Could you check a few things on this model? Use its own coordinates, in mm. Face numbers are marked on the shaded views. A direction names the side the tool comes from. Coordinates: 2 decimals unless noted, no trailing zeros. Write each loop counter-clockwise with the first axis right and the second up, starting at its lowest first coordinate (ties: lowest second). Pieces come first, ordered by that corner, then holes.
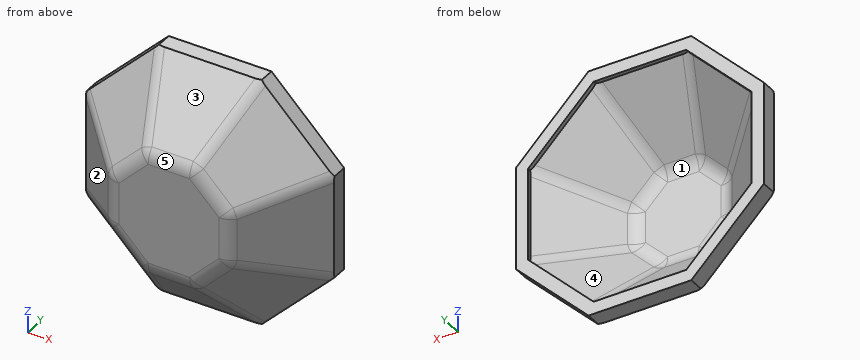
Autodesk Inventor part; units mm, degrees
ref_plane "YZ Plane" through (0, 0, 0) normal (1, 0, 0) x (0, 1, 0)
ref_plane "XZ Plane" through (0, 0, 0) normal (0, 1, 0) x (-1, 0, 0)
ref_plane "XY Plane" through (0, 0, 0) normal (0, 0, 1) x (1, 0, 0)
sketch "Sketch1" plane through (0, 0, 0) normal (0, 1, 0) x (-1, 0, 0)
  line L0 (-62.7534, -151.5) -> (-151.5, -62.7534)
  line L1 (-151.5, -62.7534) -> (-151.5, 62.7534)
  line L2 (-151.5, 62.7534) -> (-62.7534, 151.5)
  line L3 (-62.7534, 151.5) -> (62.7534, 151.5)
  line L4 (62.7534, 151.5) -> (151.5, 62.7534)
  line L5 (151.5, 62.7534) -> (151.5, -62.7534)
  line L6 (151.5, -62.7534) -> (62.7534, -151.5)
  line L7 (62.7534, -151.5) -> (-62.7534, -151.5)
  point P0 (0, 0)
  point P1 (0, 0)
  dimension "d0" = 303
extrude "Extrusion1" add sketch "Sketch1" along normal blind 100
sketch "Sketch2" plane through (0, 100, 0) normal (0, 1, 0) x (1, 0, 0)
  line L0 (-136.5, 56.5402) -> (-56.5402, 136.5)
  line L1 (-56.5402, 136.5) -> (56.5402, 136.5)
  line L2 (56.5402, 136.5) -> (136.5, 56.5402)
  line L3 (136.5, 56.5402) -> (136.5, -56.5402)
  line L4 (136.5, -56.5402) -> (56.5402, -136.5)
  line L5 (56.5402, -136.5) -> (-56.5402, -136.5)
  line L6 (-56.5402, -136.5) -> (-136.5, -56.5402)
  line L7 (-136.5, -56.5402) -> (-136.5, 56.5402)
  point P0 (0, 0)
  point P1 (0, 0)
  dimension "d3" = 273
extrude "Extrusion2" cut sketch "Sketch2" against normal blind 85
chamfer "Chamfer1" distance 80 angle 45 8 edges at (0, 15, 136.5) (96.5201, 15, 96.5201) (-96.5201, 15, 96.5201) (136.5, 15, 0) (96.5201, 15, -96.5201) (0, 15, -136.5) (-96.5201, 15, -96.5201) (-136.5, 15, 0)
chamfer "Chamfer2" distance 80 angle 45 8 edges at (-107.1267, 0, -107.1267) (0, 0, -151.5) (-151.5, 0, 0) (107.1267, 0, -107.1267) (151.5, 0, 0) (107.1267, 0, 107.1267) (0, 0, 151.5) (-107.1267, 0, 107.1267)
fillet "Fillet1" radius 25 16 edges at (46.1848, 40, 111.5) (111.5, 40, 46.1848) (111.5, 40, -46.1848) (-46.1848, 40, 111.5) (-111.5, 40, 46.1848) (46.1848, 40, -111.5) (-46.1848, 40, -111.5) (-111.5, 40, -46.1848) (-50.5581, 0, -50.5581) (0, 0, -71.5) (-71.5, 0, 0) (-50.5581, 0, 50.5581) (0, 0, 71.5) (50.5581, 0, 50.5581) (71.5, 0, 0) (50.5581, 0, -50.5581)
fillet "Fillet2" radius 25 16 edges at (39.9716, 55, 96.5) (96.5, 55, 39.9716) (96.5, 55, -39.9716) (-39.9716, 55, 96.5) (39.9716, 55, -96.5) (-39.9716, 55, -96.5) (-96.5, 55, -39.9716) (-96.5, 55, 39.9716) (-56.5, 15, 0) (-39.9515, 15, 39.9515) (-39.9515, 15, -39.9515) (0, 15, -56.5) (0, 15, 56.5) (39.9515, 15, 39.9515) (56.5, 15, 0) (39.9515, 15, -39.9515)
sketch "Sketch3" plane through (62.7534, 81.319, -151.5) normal (0.7071, 0, -0.7071) x (-0.7071, 0, -0.7071)
  circle A0 centre (-10, 7.5) radius 2
  point P0 (-62.7534, -81.319)
  dimension "d14" = 4
sketch "Sketch4" plane through (-62.7534, 81.319, 151.5) normal (-0.7071, 0, 0.7071) x (0.7071, 0, 0.7071)
  circle A0 centre (-115, 7.5) radius 2
  point P0 (-62.7534, -81.319)
  dimension "d15" = 4
sketch "Sketch5" plane through (62.7534, 81.319, -151.5) normal (0.7071, 0, -0.7071) x (-0.7071, 0, -0.7071)
  circle A0 centre (-62.755, 9.34) radius 2
  point P0 (-62.7534, -81.319)
  dimension "d16" = 4
sketch "Sketch6" plane through (-62.7534, 81.319, 151.5) normal (-0.7071, 0, 0.7071) x (0.7071, 0, 0.7071)
  circle A0 centre (-62.755, 9.34) radius 2
  point P0 (-62.7534, -81.319)
  dimension "d17" = 4
properties part number "trail 6.1" material "PVC, Unplasticized"
Item 1: I want a section at A-A, the plane z = 0.5. List the corners of the cut face in (x, y) for me, then the cut area to 4 significant figures.
Item 2: If I drill on line 1 along Z through (x, y) = (-96.5, 82); line 2 along X through (y, z) = (29, -58.5); line 3 along X through (y, z) = (66, -49.5), over which ranges is the centre line in solid material (lowest first)?
Item 3: Which directions (+Z, -Z, +X, -X, +Y, -Y) give clear straight access to the entire face, cutting with the end or side of a thin tool? Please do the marked faces 4 and 5.
Item 4: If we mould it in two halves opening along Z, with no side actions, what happens to the marked faces 1, 2 and 3? For each: released by +Z, released by -Z, zero draft, split by the parting line, or undercut.
Item 5: Will these pins go through, and if not, where does the flat tip stop? pin 1 Ø6 at (y, z) = (11, -74) entering from +X; pin 2 Ø10 at (x, z) = (48.5, -86) entering from -Y; pin 3 Ø12 at (x, y) = (70, 63.5) entering from +Z.
Taken from the geometry:
1. outline: (-151.5, 80) - (-78.82, 7.32) arc R25 ccw to (-61.14, 0) - (61.14, 0) arc R25 ccw to (78.82, 7.32) - (151.5, 80) - (151.5, 100) - (136.5, 100) - (136.5, 95) - (63.82, 22.32) arc R25 cw to (46.14, 15) - (-46.14, 15) arc R25 cw to (-63.82, 22.32) - (-136.5, 95) - (-136.5, 100) - (-151.5, 100) - close
1. area: 7,095 mm2
2. line 1: z = -117.75 to -78.16, 78.16 to 117.75
2. line 2: x = -83.63 to -41.2, 41.2 to 83.63
2. line 3: x = -137.5 to -102.52, 102.52 to 137.5
3. face 4: +Y
3. face 5: +Z, +X, -X, -Y
4. face 1: undercut
4. face 2: zero draft
4. face 3: released by +Z
5. pin 1: stops at x = 47.87
5. pin 2: stops at y = 18.61
5. pin 3: stops at z = 131.31
